```python
from build123d import *

# Parameters (mm, degrees)
F0_R     = 2.25
F1_DEPTH = 25


with BuildPart() as f1:
    # F0 (on Top) → F1 (new body)
    with BuildSketch(Plane.XY):
        with BuildLine():
            ThreePointArc((0, -30), (21.213203, -21.213203), (30, 0))
            ThreePointArc((30, 0), (21.213203, 21.213203), (0, 30))
            Line((0, 30), (0, 28))
            ThreePointArc((0, 28), (1.59099, 27.34099), (2.25, 25.75))
            ThreePointArc((2.25, 25.75), (1.59099, 24.15901), (0, 23.5))
            Line((0, 23.5), (0, 21.5))
            ThreePointArc((0, 21.5), (1.59099, 20.84099), (2.25, 19.25))
            ThreePointArc((2.25, 19.25), (1.59099, 17.65901), (0, 17))
            Line((0, 17), (0, 15))
            ThreePointArc((0, 15), (1.59099, 14.34099), (2.25, 12.75))
            ThreePointArc((2.25, 12.75), (1.59099, 11.15901), (0, 10.5))
            Line((0, 10.5), (0, 8.5))
            ThreePointArc((0, 8.5), (1.59099, 7.84099), (2.25, 6.25))
            ThreePointArc((2.25, 6.25), (1.59099, 4.65901), (0, 4))
            Line((0, 4), (0, 2.25))
            ThreePointArc((0, 2.25), (1.59099, 1.59099), (2.25, 0))
            ThreePointArc((2.25, 0), (1.59099, -1.59099), (0, -2.25))
            Line((0, -2.25), (0, -4))
            ThreePointArc((0, -4), (1.59099, -4.65901), (2.25, -6.25))
            ThreePointArc((2.25, -6.25), (1.59099, -7.84099), (0, -8.5))
            Line((0, -8.5), (0, -10.5))
            ThreePointArc((0, -10.5), (1.59099, -11.15901), (2.25, -12.75))
            ThreePointArc((2.25, -12.75), (1.59099, -14.34099), (0, -15))
            Line((0, -15), (0, -17))
            ThreePointArc((0, -17), (1.59099, -17.65901), (2.25, -19.25))
            ThreePointArc((2.25, -19.25), (1.59099, -20.84099), (0, -21.5))
            Line((0, -21.5), (0, -23.5))
            ThreePointArc((0, -23.5), (1.59099, -24.15901), (2.25, -25.75))
            ThreePointArc((2.25, -25.75), (1.59099, -27.34099), (0, -28))
            Line((0, -28), (0, -30))
        make_face()
        with Locations((6.66459, -24.87259)):
            Circle(F0_R, mode=Mode.SUBTRACT)
        with Locations((6.583888, -18.089083)):
            Circle(F0_R, mode=Mode.SUBTRACT)
        with Locations((12.875, -22.300154)):
            Circle(F0_R, mode=Mode.SUBTRACT)
        with Locations((18.208, -18.208)):
            Circle(F0_R, mode=Mode.SUBTRACT)
        with Locations((6.375, -11.041824)):
            Circle(F0_R, mode=Mode.SUBTRACT)
        with Locations((12.373661, -14.746356)):
            Circle(F0_R, mode=Mode.SUBTRACT)
        with Locations((5.412659, -3.125)):
            Circle(F0_R, mode=Mode.SUBTRACT)
        with Locations((11.041824, -6.375)):
            Circle(F0_R, mode=Mode.SUBTRACT)
        with Locations((22.300154, -12.875)):
            Circle(F0_R, mode=Mode.SUBTRACT)
        with Locations((16.670989, -9.625)):
            Circle(F0_R, mode=Mode.SUBTRACT)
        with Locations((18.957549, -3.342727)):
            Circle(F0_R, mode=Mode.SUBTRACT)
        with Locations((24.87259, -6.66459)):
            Circle(F0_R, mode=Mode.SUBTRACT)
        with Locations((5.412659, 3.125)):
            Circle(F0_R, mode=Mode.SUBTRACT)
        with Locations((12.75, 0)):
            Circle(F0_R, mode=Mode.SUBTRACT)
        with Locations((11.041824, 6.375)):
            Circle(F0_R, mode=Mode.SUBTRACT)
        with Locations((6.375, 11.041824)):
            Circle(F0_R, mode=Mode.SUBTRACT)
        with Locations((12.373661, 14.746356)):
            Circle(F0_R, mode=Mode.SUBTRACT)
        with Locations((18.957549, 3.342727)):
            Circle(F0_R, mode=Mode.SUBTRACT)
        with Locations((25.75, 0)):
            Circle(F0_R, mode=Mode.SUBTRACT)
        with Locations((24.87259, 6.66459)):
            Circle(F0_R, mode=Mode.SUBTRACT)
        with Locations((16.670989, 9.625)):
            Circle(F0_R, mode=Mode.SUBTRACT)
        with Locations((22.300154, 12.875)):
            Circle(F0_R, mode=Mode.SUBTRACT)
        with Locations((6.583888, 18.089083)):
            Circle(F0_R, mode=Mode.SUBTRACT)
        with Locations((12.875, 22.300154)):
            Circle(F0_R, mode=Mode.SUBTRACT)
        with Locations((6.66459, 24.87259)):
            Circle(F0_R, mode=Mode.SUBTRACT)
        with Locations((18.208, 18.208)):
            Circle(F0_R, mode=Mode.SUBTRACT)
        with BuildLine():
            Line((0, 28), (0, 30))
            ThreePointArc((0, 30), (-30, 0), (0, -30))
            Line((0, -30), (0, -28))
            ThreePointArc((0, -28), (-2.25, -25.75), (0, -23.5))
            Line((0, -23.5), (0, -21.5))
            ThreePointArc((0, -21.5), (-2.25, -19.25), (0, -17))
            Line((0, -17), (0, -15))
            ThreePointArc((0, -15), (-2.25, -12.75), (0, -10.5))
            Line((0, -10.5), (0, -8.5))
            ThreePointArc((0, -8.5), (-2.25, -6.25), (0, -4))
            Line((0, -4), (0, -2.25))
            ThreePointArc((0, -2.25), (-2.25, 0), (0, 2.25))
            Line((0, 2.25), (0, 4))
            ThreePointArc((0, 4), (-2.25, 6.25), (0, 8.5))
            Line((0, 8.5), (0, 10.5))
            ThreePointArc((0, 10.5), (-2.25, 12.75), (0, 15))
            Line((0, 15), (0, 17))
            ThreePointArc((0, 17), (-2.25, 19.25), (0, 21.5))
            Line((0, 21.5), (0, 23.5))
            ThreePointArc((0, 23.5), (-2.25, 25.75), (0, 28))
        make_face()
        with Locations((-18.208, -18.208)):
            Circle(F0_R, mode=Mode.SUBTRACT)
        with Locations((-6.66459, -24.87259)):
            Circle(F0_R, mode=Mode.SUBTRACT)
        with Locations((-12.875, -22.300154)):
            Circle(F0_R, mode=Mode.SUBTRACT)
        with Locations((-6.583888, -18.089083)):
            Circle(F0_R, mode=Mode.SUBTRACT)
        with Locations((-22.300154, -12.875)):
            Circle(F0_R, mode=Mode.SUBTRACT)
        with Locations((-16.670989, -9.625)):
            Circle(F0_R, mode=Mode.SUBTRACT)
        with Locations((-24.87259, -6.66459)):
            Circle(F0_R, mode=Mode.SUBTRACT)
        with Locations((-18.957549, -3.342727)):
            Circle(F0_R, mode=Mode.SUBTRACT)
        with Locations((-12.373661, -14.746356)):
            Circle(F0_R, mode=Mode.SUBTRACT)
        with Locations((-6.375, -11.041824)):
            Circle(F0_R, mode=Mode.SUBTRACT)
        with Locations((-11.041824, -6.375)):
            Circle(F0_R, mode=Mode.SUBTRACT)
        with Locations((-5.412659, -3.125)):
            Circle(F0_R, mode=Mode.SUBTRACT)
        with Locations((-25.75, 0)):
            Circle(F0_R, mode=Mode.SUBTRACT)
        with Locations((-24.87259, 6.66459)):
            Circle(F0_R, mode=Mode.SUBTRACT)
        with Locations((-18.957549, 3.342727)):
            Circle(F0_R, mode=Mode.SUBTRACT)
        with Locations((-16.670989, 9.625)):
            Circle(F0_R, mode=Mode.SUBTRACT)
        with Locations((-22.300154, 12.875)):
            Circle(F0_R, mode=Mode.SUBTRACT)
        with Locations((-12.75, 0)):
            Circle(F0_R, mode=Mode.SUBTRACT)
        with Locations((-11.041824, 6.375)):
            Circle(F0_R, mode=Mode.SUBTRACT)
        with Locations((-5.412659, 3.125)):
            Circle(F0_R, mode=Mode.SUBTRACT)
        with Locations((-12.373661, 14.746356)):
            Circle(F0_R, mode=Mode.SUBTRACT)
        with Locations((-6.375, 11.041824)):
            Circle(F0_R, mode=Mode.SUBTRACT)
        with Locations((-18.208, 18.208)):
            Circle(F0_R, mode=Mode.SUBTRACT)
        with Locations((-12.875, 22.300154)):
            Circle(F0_R, mode=Mode.SUBTRACT)
        with Locations((-6.583888, 18.089083)):
            Circle(F0_R, mode=Mode.SUBTRACT)
        with Locations((-6.66459, 24.87259)):
            Circle(F0_R, mode=Mode.SUBTRACT)
    extrude(amount=F1_DEPTH)


solid = f1.part
```
Can you work these out from the model? Positions are in its coordinate system, mm. Coordinates: 2 decimals unless noted, no trailing zeros. Write each loop counter-clockwise with the first axis right and the second up, starting at its lowest first coordinate (ties: lowest second). Pieces come first, ordered by that corner, then holes. Notation, with made-up numbers: (47, -6.5) - (81, -6.5) arc R26 cw to (81, 10.5) - close; hole circle Ø3 at (72, -10.5). An arc over 180 degrees is marked (long way). Return JSON: item names as keys, results as strings.
Q1. I'm going to push flat-ended pins straight in: pin 1 Ø12 at (y, z) = (-14.5, 21.5) entering from +X; pin 2 Ø2.5 at (x, y) = (-12.75, 0) entering from -Z; pin 3 Ø1 at (x, z) = (-19.5, 12.5) entering from +Y; pin 4 Ø8 at (x, z) = (7.5, 17) entering from -Y. Where does each tip first touch, or does it pass through?
Computed values:
{"pin 1": "stops at x = 28.77", "pin 2": "passes through", "pin 3": "stops at y = 23.22", "pin 4": "stops at y = -29.8"}
Q2. Please list where these lines run through material, in increasing order: L1, parallel to X at y = 17.5, z = 15.75; L2, parallel to Y at x = 15.5, z = 2.25; L3, parallel to X at y = 19.5, z = 17. Write a range as from..to.
Computed values:
{"L1": "x = -24.37..-20.34, -16.07..-8.76, -4.41..-1.41, 1.41..4.41, 8.76..16.07, 20.34..24.37", "L2": "y = -25.69..-11.55, -7.7..7.7, 11.55..25.69", "L3": "x = -22.8..-20.05, -16.37..-8.34, -4.83..-2.24, 2.24..4.83, 8.34..16.37, 20.05..22.8"}
Q3. If we section it at A-A (x = -25.75): Please give me the cut outline in (y, z).
Computed values:
{"outline": "(-15.39, 0) - (-8.74, 0) - (-8.74, 25) - (-15.39, 25) - close; (-4.59, 0) - (-2.25, 0) - (-2.25, 25) - (-4.59, 25) - close; (2.25, 0) - (4.59, 0) - (4.59, 25) - (2.25, 25) - close; (8.74, 0) - (15.39, 0) - (15.39, 25) - (8.74, 25) - close"}
Q4. If we section it at B-B (z = 8): Count the separate pieces of the cut face and the enclosed holes in it, then the cut area to 3 significant figures.
Computed values:
{"separate pieces": "1", "enclosed holes": "61", "area": "1,860 mm2"}
